from build123d import *

# Parameters (mm, degrees)
F1_DEPTH  = 50.8
F2_W      = 3.175
F2_H      = 22.225
F3_DEPTH  = 135.1421026655
F5_W      = 101.6
F5_H      = 0.0254
F6_DEPTH  = 0.254
F8_DEPTH  = 101.601
F9_W      = 0.0254
F9_H      = 124.7511431575
F9_H_2    = 118.2847470045
F9_H_3    = 108.944401145
F9_H_4    = 108.2259044051
F10_DEPTH = 0.254


with BuildPart() as f1:
    # F0 (on Right) → F1 (new body, symmetric)
    with BuildSketch(Plane.YZ):
        Polygon((0, -139.7), (0, 0), (-95.25, 0), (-95.25, -73.0052319855), align=None)
    extrude(amount=F1_DEPTH, both=True)

    # F2 (on face) → F3 (cut, up to face)
    with BuildSketch(Plane.XY):
        with Locations((-36.5125, -19.05)):
            Rectangle(F2_W, F2_H)
        with Locations((-14.2875, -19.05)):
            Rectangle(F2_W, F2_H)
        with Locations((14.2875, -19.05)):
            Rectangle(F2_W, F2_H)
        with Locations((36.5125, -19.05)):
            Rectangle(F2_W, F2_H)
    extrude(amount=-F3_DEPTH, mode=Mode.SUBTRACT)

    # F5 (on face) → F6 (cut)
    with BuildSketch(Plane.XY):
        with Locations((0, -19.0627)):
            Rectangle(F5_W, F5_H)
        with Locations((0, -38.1127)):
            Rectangle(F5_W, F5_H)
        with Locations((0, -57.1627)):
            Rectangle(F5_W, F5_H)
    extrude(amount=-F6_DEPTH, mode=Mode.SUBTRACT)

    # F7 (on face) → F8 (cut, through all)
    with BuildSketch(Plane.YZ.offset(50.8)):
        Polygon((-105.2813167576, -79.797580018), (-85.5495216963, -79.797580018), (-36.5125, 0), (-105.2813167576, 0), align=None)
    extrude(amount=-F8_DEPTH, mode=Mode.SUBTRACT)

    # F9 (on face) → F10 (cut)
    with BuildSketch(Plane.YZ.offset(50.8)):
        with Locations((-19.0627, -62.3755715787)):
            Rectangle(F9_W, F9_H)
        with Locations((-38.1127, -59.1423735023)):
            Rectangle(F9_W, F9_H_2)
        with Locations((-57.1627, -54.4722005725)):
            Rectangle(F9_W, F9_H_3)
        with Locations((-76.2127, -54.1129522026)):
            Rectangle(F9_W, F9_H_4)
    extrude(amount=-F10_DEPTH, mode=Mode.SUBTRACT)


solid = f1.part
Can you work these out from the model? Positions are in its coordinate system, mm. A direction names the side the tool comes from. Give positions to 0.01 mm unless a question says otherwise; leave off trailing zeros. Loops run counter-clockwise (first coordinate to the right, second up) from the corner with the lowest first, then second, coordinate; pieces in that order, holes last. Notation, with made-up numbers: (52, 37) - (105, 37) arc R13 ccw to (105, 59) - close; hole circle Ø10 at (87.5, -24.5). An arc over 180 degrees is marked (long way). One line per item, written item: value.
(1) If we section it at B-B, the plane z = -95: State how many separate pieces and enclosed holes the cut face has, plus the area to 3 significant figures.
Verdict:
separate pieces: 1
enclosed holes: 4
area: 6,200 mm^2
(2) On a 3-axis mill with a long thin cutter (end or side, diameter ignored), from which of +Z, -Z, +X, -X, +Y, -Y can I reach the whole of each face in a straight line? I mean faces 1 (the face through (-12.7, -19, -66)), 2 (the face through (1, -9, 0)). Say none if no direction works.
Verdict:
face 1: +Z, -Z
face 2: +Z, +X, -X, +Y, -Y
(3) I need wall thicknesses on line 1 along X through (y, z) = (-18.5, -101) (3 decimals); line 2 along Y through (x, z) = (31, -75); line 3 along Z through (x, y) = (-34, -35). Which ranges of each line are inside material? Lowest first, please.
Verdict:
line 1: -50.8 to -38.1, -34.925 to -15.875, -12.7 to 12.7, 15.875 to 34.925, 38.1 to 50.8
line 2: -82.6 to 0
line 3: -115.19 to 0
(4) I'm going to push flat-ended pins straight in: pin 1 (1.6 mm diameter, centred on x = -14.5, z = -54.5, fed in from -Y); pin 2 (8 mm diameter, centred on x = -3.5, y = -69.5, fed in from -Z); pin 3 (1 mm diameter, centred on x = 22, z = -122, fed in from +Y); pin 4 (1 mm diameter, centred on x = 36, z = -45.5, fed in from -Y). Where does each tip first touch, or does it pass through?
Verdict:
pin 1: y = -70.5
pin 2: z = -93.84
pin 3: y = 0
pin 4: y = -64.78
(5) If we section it at A-A, the plane y = -11: List the corners of the cut face in (x, z) for me (3 decimals).
Verdict:
outline: (-50.8, -131.998) - (-38.1, -131.998) - (-38.1, 0) - (-50.8, 0) - close; (-34.925, -131.998) - (-15.875, -131.998) - (-15.875, 0) - (-34.925, 0) - close; (-12.7, -131.998) - (12.7, -131.998) - (12.7, 0) - (-12.7, 0) - close; (15.875, -131.998) - (34.925, -131.998) - (34.925, 0) - (15.875, 0) - close; (38.1, -131.998) - (50.8, -131.998) - (50.8, 0) - (38.1, 0) - close
